Geometry check sheet. Reference: drawing and pictorial views, mm from the part's lowest x, y, z. A direction names the side the tool comes from. Round coordinates to 2 decimals unless told otherwise and drop trailing zeros. Write each loop counter-clockwise with the first axis right and the second up, starting at its lowest first coordinate (ties: lowest second). Pieces come first, ordered by that corner, then holes. Notation, with made-up numbers: M 1.5,-37 L 25.5,-37 A14 ccw 25.5,-29 Z; hole C -15.5,-4.5 d2. An arc over 180 degrees is marked long. Use a Markdown table: item, result. Add a question column.
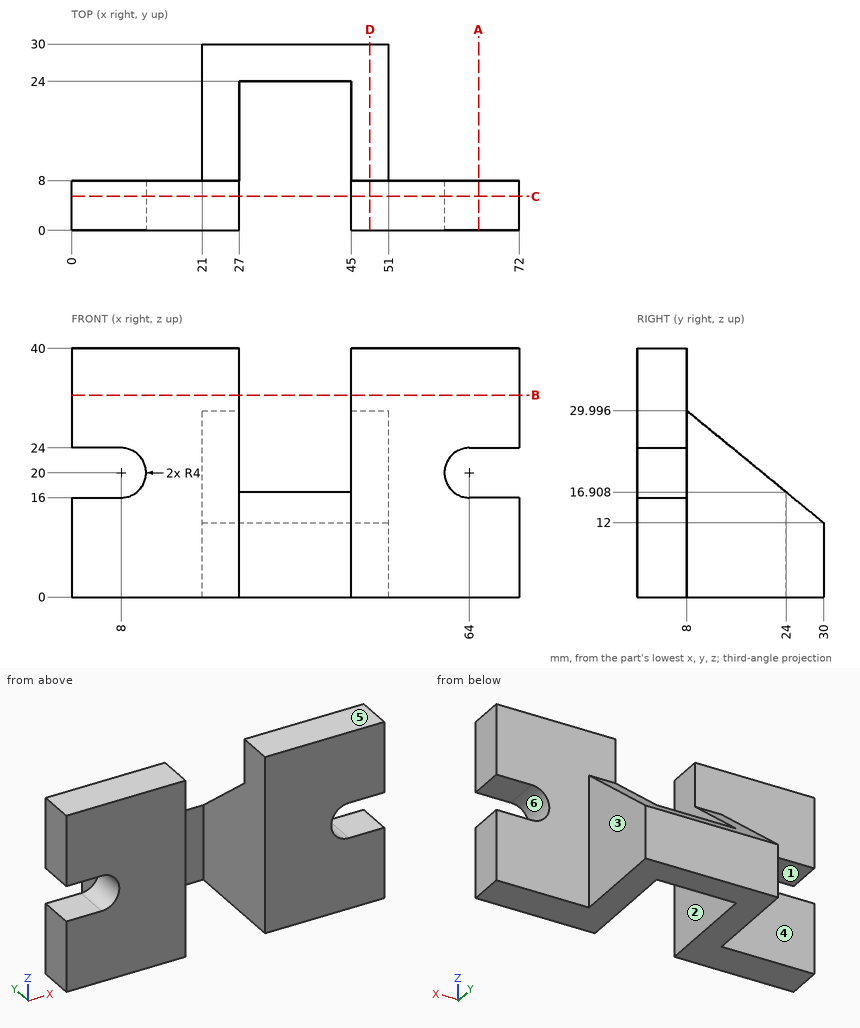
1. Cross-section at D-D on x = 48. Enter the section's corners in (y, z).
2. Cross-section at A-A on x = 65.5. Enter the section's corners in (y, z).
3. Cross-section at B-B on z = 32.5. Enter the section's corners in (x, y).
4. Depth check by flat-ended pin: pin 1 Ø1.5 at (y, z) = (21, 15.5) entering from -X; pin 2 Ø3 at (x, y) = (44, 26.5) entering from +Z; pin 3 Ø3 at (x, z) = (35.5, 6.5) entering from -Y; pin 4 Ø5 at (x, y) = (36, 20.5) entering from -Z. Enter the tip coordinate at first touch or a pass-through.
5. Scan lines: line 1 along X through (y, z) = (7.5, 27.5); line 2 along X through (y, z) = (17.5, 14.5); line 3 along Y through (x, z) = (25, 30). Record each from-to range of solid material in increasing order. Write a range as from..to.
6. Access from +Z, -Z, +X, -X, +Y, -Y to the whole of each face (thin tool, end or side, straight path). Record for the marked faces 1, 2 and 3.
7. Cross-section at C-C on y = 5.5. Enter the section's corners in (x, z), plus the area to 3 significant figures.
8. Release check for a two-part mould opening along Z. For the marked faces 4, 5 and 6 record: +Z half, -Z half, draft (parallel to the pull), parting line (faces both ways), or undercut.
Answer:
| question | item | result |
|---|---|---|
| 1 | outline | M 0,0 L 30,0 L 30,12 L 8,30 L 8,40 L 0,40 Z |
| 2 | outline | M 0,0 L 8,0 L 8,16 L 0,16 Z; M 0,24 L 8,24 L 8,40 L 0,40 Z |
| 3 | outline | M 0,0 L 27,0 L 27,8 L 0,8 Z; M 45,0 L 72,0 L 72,8 L 45,8 Z |
| 4 | pin 1 | stops at x = 21 |
| 4 | pin 2 | stops at z = 16.09 |
| 4 | pin 3 | stops at y = 24 |
| 4 | pin 4 | passes through |
| 5 | line 1 | x = 0..27, 45..72 |
| 5 | line 2 | x = 21..27, 45..51 |
| 5 | line 3 | y = 0..8 |
| 6 | face 1 | -X, +Y, -Y |
| 6 | face 2 | +Z, -Z, -Y |
| 6 | face 3 | +Z, -Z, +X, +Y |
| 7 | outline | M 0,0 L 27,0 L 27,40 L 0,40 L 0,24 L 8,24 A4 cw 8,16 L 0,16 Z; M 45,0 L 72,0 L 72,16 L 64,16 A4 cw 64,24 L 72,24 L 72,40 L 45,40 Z |
| 7 | area | 1,980 mm^2 |
| 8 | face 4 | draft |
| 8 | face 5 | +Z half |
| 8 | face 6 | undercut |
